Could you check a few things on this model? Use its own coordinates, in mm. A direction names the side the tool comes from. Round coordinates to 2 decimals unless told otherwise and drop trailing zeros. Loops run counter-clockwise (first coordinate to the right, second up) from the corner with the lowest first, then second, coordinate; pieces in that order, holes last. Notation, with made-up numbers: (72.25, -40) -> (80.25, -40) arc R9 cw to (80.25, -34) -> close; hole circle Ø8 at (52, -34). An arc over 180 degrees is marked (long way). One line per item, written item: value.
Autodesk Inventor part; units mm, degrees
ref_plane "YZ Plane" through (0, 0, 0) normal (1, 0, 0) x (0, 1, 0)
ref_plane "XZ Plane" through (0, 0, 0) normal (0, 1, 0) x (-1, 0, 0)
ref_plane "XY Plane" through (0, 0, 0) normal (0, 0, 1) x (1, 0, 0)
sketch "Skizze1" plane through (0, 0, 0) normal (0, 1, 0) x (-1, 0, 0)
  line L0 (32.3571, 6.1813) -> (-27.6429, 6.1813)
  line L1 (-27.6429, -23.8187) -> (32.3571, -23.8187)
  line L2 (32.3571, -3.8187) -> (22.3571, -3.8187)
  line L3 (22.3571, -3.8187) -> (22.3571, -13.8187)
  line L4 (22.3571, -13.8187) -> (32.3571, -13.8187)
  line L5 (-17.6429, -3.8187) -> (-27.6429, -3.8187)
  line L6 (-27.6429, -13.8187) -> (-17.6429, -13.8187)
  line L7 (-17.6429, -13.8187) -> (-17.6429, -3.8187)
  line L8 (-27.6429, 6.1813) -> (-27.6429, -3.8187)
  line L9 (-27.6429, -13.8187) -> (-27.6429, -23.8187)
  line L10 (32.3571, -23.8187) -> (32.3571, -13.8187)
  line L11 (32.3571, -3.8187) -> (32.3571, 6.1813)
  point P0 (0, 0)
  dimension "d0" = 30
  dimension "d1" = 60
  dimension "d2" = 10
  dimension "d3" = 10
  dimension "d4" = 10
  dimension "d6" = 10
  dimension "d7" = 10
  dimension "d10" = 10
extrude "Extrusion1" add sketch "Skizze1" along normal blind 10
properties part number "KabelBoxPlatteKurz"
(1) If we section it at C-C, the plane z = -5.75: Please give me the cut outline in (x, y), then the cut area to 3 significant figures.
Recorded:
outline: (-22.36, 0) -> (17.64, 0) -> (17.64, 10) -> (-22.36, 10) -> close
area: 400 mm²
(2) Thinking about a two-plate mould opening in Z: for faces 1 (the face through (-2, 0, -9)), 2 (the face through (-3, 5, 6.181)), 3 (the face through (-27, 5, -3.819)), which applies, released by +Z, released by -Z, zero draft, split by the parting line, or undercut?
Recorded:
face 1: zero draft
face 2: released by +Z
face 3: undercut
(3) If I drill on L1, parallel to Z at x = 19.5, y = 8.75; L2, parallel to X at y = 9, z = -13, over which ranges is the centre line in solid material (lowest first)?
Recorded:
L1: -23.82 to -13.82, -3.82 to 6.18
L2: -22.36 to 17.64
(4) If we section it at A-A, the plane x = -26: Please give me the cut outline in (y, z).
Recorded:
outline: (0, -23.82) -> (10, -23.82) -> (10, -13.82) -> (0, -13.82) -> close; (0, -3.82) -> (10, -3.82) -> (10, 6.18) -> (0, 6.18) -> close
(5) If we section it at B-B, the plane y = 3: Please give me the cut outline in (x, z).
Recorded:
outline: (-32.36, -23.82) -> (27.64, -23.82) -> (27.64, -13.82) -> (17.64, -13.82) -> (17.64, -3.82) -> (27.64, -3.82) -> (27.64, 6.18) -> (-32.36, 6.18) -> (-32.36, -3.82) -> (-22.36, -3.82) -> (-22.36, -13.82) -> (-32.36, -13.82) -> close
(6) For faces 4 (the face through (23, 5, -13.819)), 5 (the face through (-22.357, 5, -9)), 6 (the face through (-32.357, 5, -19)), which set-ups out of +Z, -Z, +X, -X, +Y, -Y let a thin tool reach every point of the face, with its end or its side?
Recorded:
face 4: +X, +Y, -Y
face 5: -X, +Y, -Y
face 6: +Z, -Z, -X, +Y, -Y
